Check sheet for the modelled part. Datum: model origin and axes. Units: mm. A direction names the side the tool comes from. Round coordinates to 2 decimals unless told otherwise and drop trailing zeros. Order: outer loops, then holes, each group sorted by start corner. A loop starts at its lowest first (then second) coordinate and runs counter-clockwise, first axis right, second up. Notation, with made-up numbers: (88.25, -23) -> (103.25, -23) arc R20 cw to (103.25, -1) -> close; hole circle Ø1 at (33, -30). An arc over 180 degrees is marked (long way). Answer in a Markdown table with one row per item.
from build123d import *

# Parameters (mm, degrees)
BOSS_EXTRUDE2_DEPTH = 4
CUT_EXTRUDE1_DEPTH  = 4
SKETCH4_R           = 1.35
CUT_EXTRUDE2_DEPTH  = 4
SKETCH6_W           = 24
SKETCH6_H           = 3
CUT_EXTRUDE3_DEPTH  = 4


with BuildPart() as part:
    # Sketch1 → Boss-Extrude2 (new body)
    with BuildSketch(Plane.XY):
        Polygon((-105.5, 0), (-48.5, 0), (-48.5, -7), (-26.5, -7), (-26.5, 0), (31.5, 0), (31.5, -7), (53.5, -7), (53.5, 0), (110.5, 0), (110.5, -7), (117.5, -7), (117.5, 0), (117.5, 10), (82.5, 41), (62.5, 41), (62.5, 46), (47.5, 46), (47.5, 41), (-2.5, 41), (-2.5, 46), (-22.5, 46), (-22.5, 41), (-72.5, 41), (-72.5, 46), (-92.5, 46), (-92.5, 41), (-117.5, 41), (-117.5, 0), (-117.5, -7), (-105.5, -7), align=None)
    extrude(amount=BOSS_EXTRUDE2_DEPTH)

    # Sketch2 → Cut-Extrude1 (cut)
    with BuildSketch(Plane.XY.offset(4)):
        Polygon((-71.5, 20), (-71.5, 24.3), (-57.5, 24.3), (-57.5, 15.7), (-71.5, 15.7), align=None)
        Polygon((52.5, 20), (52.5, 24.3), (66.5, 24.3), (66.5, 15.7), (52.5, 15.7), align=None)
    extrude(amount=-CUT_EXTRUDE1_DEPTH, mode=Mode.SUBTRACT)

    # Sketch4 → Cut-Extrude2 (cut)
    with BuildSketch(Plane.XY.offset(4)):
        with Locations((-38.25, 37.55)):
            Circle(SKETCH4_R)
        with Locations((-90.75, 37.55)):
            Circle(SKETCH4_R)
        with Locations((-90.75, 3.45)):
            Circle(SKETCH4_R)
        with Locations((-38.25, 3.45)):
            Circle(SKETCH4_R)
        with Locations((27, 37.55)):
            Circle(SKETCH4_R)
        with Locations((79.5, 37.55)):
            Circle(SKETCH4_R)
        with Locations((79.5, 3.45)):
            Circle(SKETCH4_R)
        with Locations((27, 3.45)):
            Circle(SKETCH4_R)
    extrude(amount=-CUT_EXTRUDE2_DEPTH, mode=Mode.SUBTRACT)

    # Sketch6 → Cut-Extrude3 (cut)
    with BuildSketch(Plane.XY.offset(4)):
        with Locations((-64.5, 32.65)):
            Rectangle(SKETCH6_W, SKETCH6_H)
        with Locations((-64.5, 7.85)):
            Rectangle(SKETCH6_W, SKETCH6_H)
        with Locations((59.5, 35.15)):
            Rectangle(SKETCH6_W, SKETCH6_H)
        with Locations((59.5, 7.85)):
            Rectangle(SKETCH6_W, SKETCH6_H)
        Polygon((-83.5, 20), (-83.5, 26), (-86.5, 26), (-86.5, 14), (-83.5, 14), align=None)
        Polygon((-45.5, 20), (-45.5, 26), (-42.5, 26), (-42.5, 14), (-45.5, 14), align=None)
        Polygon((40.5, 20), (40.5, 26), (37.5, 26), (37.5, 14), (40.5, 14), align=None)
        Polygon((78.5, 20), (78.5, 26), (81.5, 26), (81.5, 14), (78.5, 14), align=None)
    extrude(amount=-CUT_EXTRUDE3_DEPTH, mode=Mode.SUBTRACT)


solid = part.part
Item 1: Cross-section at D-D (x = 11). Record the boundary of the cut face in (y, z), and give its area (3 significant figures).
Result sheet:
| item | result |
|---|---|
| outline | (0, 0) -> (41, 0) -> (41, 4) -> (0, 4) -> close |
| area | 164 mm^2 |
Item 2: Depth check by flat-ended pin: P1, Ø1.2, axis at x = -66, z = 2.5, coming from the -Y side; P2, Ø1.2, axis at x = 75.5, z = 1, coming from the +Y side. Enter the tip coordinate at first touch or a pass-through.
Result sheet:
| item | result |
|---|---|
| P1 | stops at y = 0 |
| P2 | stops at y = 41 |
Item 3: Mould release check, pull along Y, two halves, no side actions. Record for faces 1 (the flat face through (31.5, -3, 2)), 2 (the flat face through (114, -7, 2)), 3 (the flat face through (66.5, 20, 2)): pulls with the +Y half, pulls with the -Y half, needs draft (parallel to the pull), parting line crosses it, or undercut.
Result sheet:
| item | result |
|---|---|
| face 1 | needs draft |
| face 2 | pulls with the -Y half |
| face 3 | undercut |
Item 4: Scan lines: line 1 (Y direction, x = 51, z = 3.65); line 2 (Y direction, x = 65.5, z = 1.55); line 3 (X direction, y = 8, z = 0.95). Record each from-to range of solid material in increasing order. Write a range as [from, to].
Result sheet:
| item | result |
|---|---|
| line 1 | y = [-7, 6.35], [9.35, 33.65], [36.65, 46] |
| line 2 | y = [0, 6.35], [9.35, 15.7], [24.3, 33.65], [36.65, 41] |
| line 3 | x = [-117.5, -76.5], [-52.5, 47.5], [71.5, 117.5] |
Item 5: Cross-section at C-C (z = 2.4). State how many separate pieces and enclosed holes the cut face has, and give its area (3 significant figures).
Result sheet:
| item | result |
|---|---|
| separate pieces | 1 |
| enclosed holes | 18 |
| area | 9,090 mm^2 |
Item 6: Cross-section at B-B (x = -68). Record the boundary of the cut face in (y, z).
Result sheet:
| item | result |
|---|---|
| outline | (0, 0) -> (6.35, 0) -> (6.35, 4) -> (0, 4) -> close; (9.35, 0) -> (15.7, 0) -> (15.7, 4) -> (9.35, 4) -> close; (24.3, 0) -> (31.15, 0) -> (31.15, 4) -> (24.3, 4) -> close; (34.15, 0) -> (41, 0) -> (41, 4) -> (34.15, 4) -> close |
Item 7: Cross-section at A-A (y = -2.5). Record the boundary of the cut face in (x, z).
Result sheet:
| item | result |
|---|---|
| outline | (-117.5, 0) -> (-105.5, 0) -> (-105.5, 4) -> (-117.5, 4) -> close; (-48.5, 0) -> (-26.5, 0) -> (-26.5, 4) -> (-48.5, 4) -> close; (31.5, 0) -> (53.5, 0) -> (53.5, 4) -> (31.5, 4) -> close; (110.5, 0) -> (117.5, 0) -> (117.5, 4) -> (110.5, 4) -> close |
Item 8: Set-up check for faces 4 (the flat face through (59, 36.65, 2)), 5 (the flat face through (73, 41, 2)), 6 (the flat face through (2, 0, 2)), 7 (the flat face through (-117.5, 17, 2)), 8 (the flat face through (-22.5, 44, 2)): record each of +Z, -Z, +X, -X, +Y, -Y from which the full face is reachable in a straight line by a thin tool's end or side.
Result sheet:
| item | result |
|---|---|
| face 4 | +Z, -Z |
| face 5 | +Z, -Z, +X, +Y |
| face 6 | +Z, -Z, -Y |
| face 7 | +Z, -Z, -X, +Y, -Y |
| face 8 | +Z, -Z, +Y |
